For this review, take the finished solid that the model builds, in its own axes (mm). Give positions to 0.01 mm unless a question says otherwise; leave off trailing zeros. Order: outer loops, then holes, each group sorted by start corner. A loop starts at its lowest first (then second) coordinate and runs counter-clockwise, first axis right, second up. Notation, with made-up numbers: (-1.5, 21) - (32.5, 21) arc R28 ccw to (32.5, 56) - close; hole circle Ø6 at (27, 41.25). An arc over 180 degrees is marked (long way). One line per item, written item: value.
Autodesk Inventor part; units mm, degrees
ref_plane "YZ Plane" through (0, 0, 0) normal (1, 0, 0) x (0, 1, 0)
ref_plane "XZ Plane" through (0, 0, 0) normal (0, 1, 0) x (-1, 0, 0)
ref_plane "XY Plane" through (0, 0, 0) normal (0, 0, 1) x (1, 0, 0)
sketch "Sketch1" plane through (0, 0, 0) normal (0, 1, 0) x (-1, 0, 0)
  line L0 (-28, 42.5) -> (28, 42.5)
  line L1 (28, 42.5) -> (28, -42.5)
  line L2 (28, -42.5) -> (-28, -42.5)
  line L3 (-28, -42.5) -> (-28, 42.5)
  point P0 (0, 0)
  point P1 (28, 0)
  point P2 (0, 42.5)
  dimension "d0" = 85
  dimension "d1" = 56
extrude "Extrusion1" add sketch "Sketch1" along normal blind 18
sketch "Sketch2" plane through (0, 18, 0) normal (0, 1, 0) x (1, 0, 0)
  circle A0 centre (-24.5, -39) radius 1.375
  circle A1 centre (24.5, -39) radius 1.375
  circle A2 centre (24.5, 19) radius 1.375
  circle A3 centre (-24.5, 19) radius 1.375
  line L0 (-28, 42.5) -> (-28, -42.5)
  line L1 (28, 42.5) -> (28, -42.5)
  line L2 (-28, -42.5) -> (28, -42.5)
  point P0 (0, 0)
  dimension "d4" = 3.5
  dimension "d5" = 3.5
  dimension "d6" = 58
  dimension "d7" = 2.75
  dimension "d8" = 3.5
extrude "Extrusion2" cut sketch "Sketch2" against normal through all
fillet "Fillet1" radius 3 4 edges at (28, 9, -42.5) (-28, 9, -42.5) (28, 9, 42.5) (-28, 9, 42.5)
equation "\"d0\" = Rpi_width"
equation "\"d1\" = Rpi_heigth"
equation "\"d4\" = Rpi_hole_distance_wall"
equation "\"d5\" = d4"
equation "\"d6\" = Rpi_hole_distance_between"
equation "\"d7\" = Rpi_hole_diameter"
equation "\"d8\" = d4"
equation "\"d11\" = Rpi_corner_radius"
equation "\"Rpi_hole_diameter\" = 2.75"
equation "\"Rpi_hole_distance_wall\" = 3.5"
equation "\"Rpi_hole_distance_between\" = 58"
equation "\"Rpi_width\" = 85"
equation "\"Rpi_heigth\" = 56"
equation "\"Rpi_corner_radius\" = 3"
properties part number "RaspberryPi_Placeholder"
(1) Wall thickness on line 1 (Z direction, x = 24.5, y = 9.5) (3 decimals); line 2 (X direction, y = 5.25, z = 39) (3 decimals): over which ranges is each line inside the solid? List them lowest first. Write a range as from..to.
Answers below:
line 1: z = -42.5..-20.375, -17.625..37.625, 40.375..42.5
line 2: x = -28..-25.875, -23.125..23.125, 25.875..28
(2) Take a section at A-A (z = -19). Write out the cut boundary in (x, y) (3 decimals), then the cut area to 3 significant figures.
Answers below:
outline: (-28, 0) - (-25.875, 0) - (-25.875, 18) - (-28, 18) - close; (-23.125, 0) - (23.125, 0) - (23.125, 18) - (-23.125, 18) - close; (25.875, 0) - (28, 0) - (28, 18) - (25.875, 18) - close
area: 909 mm^2
(3) Draft analysis for pull direction X (two halves, no side actions). For faces 1 (the face through (27.1, 9.13, 41.64)), 2 (the face through (0, 18, 1)), 3 (the face through (-25.513, 9.126, 38.071)), state which applies: pulls with the +X half, pulls with the -X half, needs draft (parallel to the pull), parting line crosses it, or undercut.
Answers below:
face 1: pulls with the +X half
face 2: needs draft
face 3: undercut
(4) For P1, Ø3, axis at x = 24.5, z = -19, coming from the +Y side, flat-tipped, find the tip position at first contact; note if it passes through.
Answers below:
P1: stops at y = 18
